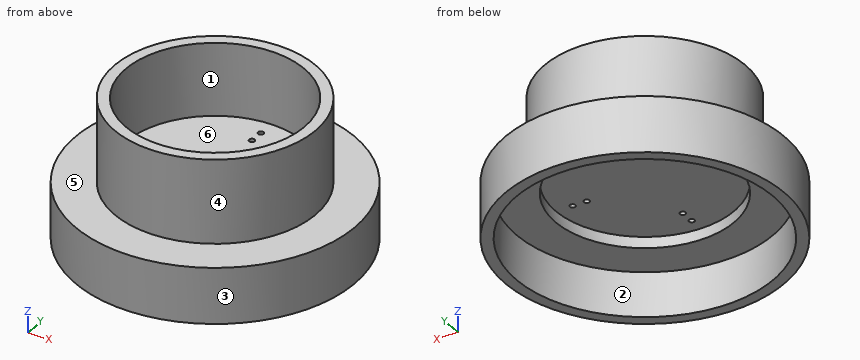
```python
from build123d import *

# Parameters (mm, degrees)
F0_R     = 18
F1_DEPTH = 15
F2_T     = -2
F3_R     = 25
F4_DEPTH = 10
F5_T     = -2
F7_D     = 1
F8_D     = 1
F9_D     = 1
F10_D    = 1
F11_D    = 1
F12_D    = 1
F13_D    = 1
F14_D    = 1


with BuildPart() as f1:
    # F0 (on Top) → F1 (new body)
    with BuildSketch(Plane.XY):
        Circle(F0_R)
    extrude(amount=-F1_DEPTH)

    # F2
    f2_openings = [f1.faces().sort_by_distance(p)[0] for p in [
        (0, 0, 0),
    ]]
    offset(amount=F2_T, openings=f2_openings)

    # F3 (on face) → F4 (join)
    with BuildSketch(Plane(origin=(0, 0, -15), x_dir=(1, 0, 0), z_dir=(0, 0, -1))):
        Circle(F3_R)
    extrude(amount=F4_DEPTH)

    # F5
    f5_openings = [f1.faces().sort_by_distance(p)[0] for p in [
        (0, 0, -25),
    ]]
    offset(amount=F5_T, openings=f5_openings, kind=Kind.INTERSECTION)

    # F7 (through all)
    with Locations(Plane(origin=(0, 0, -15), x_dir=(1, 0, 0), z_dir=(0, 0, -1))):
        with Locations((0, -13)):
            Hole(F7_D / 2)

    # F8 (through all)
    with Locations(Plane(origin=(0, 0, -15), x_dir=(1, 0, 0), z_dir=(0, 0, -1))):
        with Locations((0, -10.46)):
            Hole(F8_D / 2)

    # F9 (through all)
    with Locations(Plane(origin=(0, 0, -15), x_dir=(1, 0, 0), z_dir=(0, 0, -1))):
        with Locations((-13, 0)):
            Hole(F9_D / 2)

    # F10 (through all)
    with Locations(Plane(origin=(0, 0, -15), x_dir=(1, 0, 0), z_dir=(0, 0, -1))):
        with Locations((-10.46, 0)):
            Hole(F10_D / 2)

    # F11 (through all)
    with Locations(Plane(origin=(0, 0, -15), x_dir=(1, 0, 0), z_dir=(0, 0, -1))):
        with Locations((0, 13.3159505203)):
            Hole(F11_D / 2)

    # F12 (through all)
    with Locations(Plane(origin=(0, 0, -15), x_dir=(1, 0, 0), z_dir=(0, 0, -1))):
        with Locations((0, 10.7759505203)):
            Hole(F12_D / 2)

    # F13 (through all)
    with Locations(Plane(origin=(0, 0, -15), x_dir=(1, 0, 0), z_dir=(0, 0, -1))):
        with Locations((13, 0)):
            Hole(F13_D / 2)

    # F14 (through all)
    with Locations(Plane(origin=(0, 0, -15), x_dir=(1, 0, 0), z_dir=(0, 0, -1))):
        with Locations((10.46, 0)):
            Hole(F14_D / 2)


solid = f1.part
```
Check sheet for the modelled part. Datum: model origin and axes. Units: mm. Face numbers are marked on the shaded views. A direction names the side the tool comes from. Round coordinates to 2 decimals unless told otherwise and drop trailing zeros. Loops run counter-clockwise (first coordinate to the right, second up) from the corner with the lowest first, then second, coordinate; pieces in that order, holes last. Notation, with made-up numbers: (49, -5.5) -> (82, -5.5) arc R24 ccw to (82, 8.5) -> close; hole circle Ø1 at (44, 38). An arc over 180 degrees is marked (long way). Answer in a Markdown table with one row per item.
Q1. Sectioned sample at A-A on x = 8.5. Enter the section's corners in (y, z), then the cut area to 3 significant figures.
Data:
| item | result |
|---|---|
| outline | (-23.51, -25) -> (-21.37, -25) -> (-21.37, -17) -> (-13.56, -17) -> (-13.56, -15) -> (13.56, -15) -> (13.56, -17) -> (21.37, -17) -> (21.37, -25) -> (23.51, -25) -> (23.51, -15) -> (15.87, -15) -> (15.87, 0) -> (13.56, 0) -> (13.56, -13) -> (-13.56, -13) -> (-13.56, 0) -> (-15.87, 0) -> (-15.87, -15) -> (-23.51, -15) -> close |
| area | 198 mm^2 |
Q2. Sectioned sample at C-C on z = -4.5. Enter the section's corners in (x, y), then the cut area to 3 significant figures.
Data:
| item | result |
|---|---|
| outline | circle Ø36 at (0, 0); hole circle Ø32 at (0, 0) |
| area | 214 mm^2 |
Q3. Release check for a two-part mould opening along Y. For the marked faces 4, 5 and 6 record: released by +Y, released by -Y, zero draft, split by the parting line, or undercut.
Data:
| item | result |
|---|---|
| face 4 | split by the parting line |
| face 5 | zero draft |
| face 6 | undercut |
Q4. Thickness scan on L1, parallel to Y at x = 0, z = -2.5; L2, parallel to Y at x = 0, z = -16.2; L3, parallel to Z at x = -8, y = 18. Record the ranges inside material, lowest first.
Data:
| item | result |
|---|---|
| L1 | y = -18 to -16, 16 to 18 |
| L2 | y = -25 to -16, 16 to 25 |
| L3 | z = -17 to -15 |
Q5. Sectioned sample at D-D on y = -21. Enter the section's corners in (x, z).
Data:
| item | result |
|---|---|
| outline | (-13.56, -25) -> (-9.38, -25) -> (-9.38, -17) -> (9.38, -17) -> (9.38, -25) -> (13.56, -25) -> (13.56, -15) -> (-13.56, -15) -> close |
Q6. Set-up check for the marked faces 1, 2 and 3: record each of +Z, -Z, +X, -X, +Y, -Y from which the full face is reachable in a straight line by a thin tool's end or side.
Data:
| item | result |
|---|---|
| face 1 | +Z |
| face 2 | -Z |
| face 3 | +Z, -Z |
Q7. Go/stop test with flat-tipped pins: P1, Ø4, axis at y = -14.5, z = -3.5, coming from the +X side; P2, Ø10, axis at x = 6, y = -5, coming from the +Z side; P3, Ø5, axis at y = -16, z = -9, coming from the -X side. Record where each tip stops, or that it passes through.
Data:
| item | result |
|---|---|
| P1 | stops at x = 12.95 |
| P2 | stops at z = -13 |
| P3 | stops at x = -11.91 |
